Design review of the part built by this model. Coordinates are the model's own, in mm. A direction names the side the tool comes from. Give positions to 0.01 mm unless a question says otherwise; leave off trailing zeros. Order: outer loops, then holes, each group sorted by start corner. A loop starts at its lowest first (then second) coordinate and runs counter-clockwise, first axis right, second up.
```python
from build123d import *

# Parameters (mm, degrees)
SKETCH1_R           = 2
BOSS_EXTRUDE3_DEPTH = 12
CHAMFER2_SIZE       = 0.5
CUT_EXTRUDE1_DEPTH  = 2


with BuildPart() as part:
    # Sketch1 → Boss-Extrude3 (new body)
    with BuildSketch(Plane(origin=(0, 0, 0), x_dir=(1, 0, 0), z_dir=(0, 1, 0))):
        Circle(SKETCH1_R)
    extrude(amount=-BOSS_EXTRUDE3_DEPTH)

    # Sketch3 → Revolve2 (revolve)
    with BuildSketch(Plane.XY):
        with BuildLine():
            Line((-2, 0), (0, 0))
            Line((0, 0), (0, 2))
            Line((0, 2), (-3.517157288, 2))
            ThreePointArc((-3.517157288, 2), (-3.701933194, 1.876536686), (-3.658578644, 1.658578644))
            Line((-3.658578644, 1.658578644), (-2, 0))
        make_face()
    revolve(axis=Axis((0, -2, 0), (0, 1, 0)))

    # Chamfer2
    chamfer2_edges = [part.edges().sort_by_distance(p)[0] for p in [
        (-2, -12, 0),
    ]]
    chamfer(chamfer2_edges, length=CHAMFER2_SIZE)

    # Sketch4 → Cut-Extrude1 (cut)
    with BuildSketch(Plane(origin=(0, 2, 0), x_dir=(1, 0, 0), z_dir=(0, 1, 0))):
        Polygon((1.303085549, -1.141038146), (1.639710796, 0.557986116), (0.336625247, 1.699024262), (-1.303085549, 1.141038146), (-1.639710796, -0.557986116), (-0.336625247, -1.699024262), align=None)
    extrude(amount=-CUT_EXTRUDE1_DEPTH, mode=Mode.SUBTRACT)


solid = part.part
```
1. Take a section at B-B (z = 0). State the section outline as (x, y) points, then the cut area to 3 significant figures.
Recorded:
outline: (-3.66, 1.66) - (-2, 0) - (-2, -11.5) - (-1.5, -12) - (1.5, -12) - (2, -11.5) - (2, 0) - (3.66, 1.66) arc R0.2 ccw to (3.52, 2) - (1.53, 2) - (1.53, 0) - (-1.53, 0) - (-1.53, 2) - (-3.52, 2) arc R0.2 ccw to start
area: 53.5 mm2
2. For pin 1 (2 mm diameter, centred on y = -4, z = 2.5, fed in from +X); pin 2 (4 mm diameter, centred on x = 3, y = -2.5, fed in from -Z); pin 3 (4 mm diameter, centred on y = -4.5, z = 2, fed in from +X), all flat-tipped, find the tip position at first contact; note any pin that passes through.
Recorded:
pin 1: stops at x = 1.32
pin 2: stops at z = -1.73
pin 3: stops at x = 2
3. For line 1 along X through (y, z) = (-10, 0); line 2 along Y through (x, z) = (0, 0.25); line 3 along X through (y, z) = (-5.25, 0.75), list the stretches that pass through material, from the lowest coordinate up.
Recorded:
line 1: x = -2 to 2
line 2: y = -12 to 0
line 3: x = -1.85 to 1.85
4. Draft analysis for pull direction X (two halves, no side actions). For faces 3 (the face through (0, 0, 0)), 4 (the face through (0, -6, 2)), 5 (the face through (0, -12, 0)), state which applies: pulls with the +X half, pulls with the -X half, needs draft (parallel to the pull), parting line crosses it, or undercut.
Recorded:
face 3: undercut
face 4: parting line crosses it
face 5: needs draft
5. Take a section at A-A (x = 0). State the section outline as (y, z) points.
Recorded:
outline: (-12, -1.5) - (-11.5, -2) - (0, -2) - (1.66, -3.66) arc R0.2 ccw to (2, -3.52) - (2, -1.58) - (0, -1.58) - (0, 1.58) - (2, 1.58) - (2, 3.52) arc R0.2 ccw to (1.66, 3.66) - (0, 2) - (-11.5, 2) - (-12, 1.5) - close
6. Take a section at C-C (y = -2). State the section outline as (x, z) points, then the cut area to 3 significant figures.
Recorded:
outline: circle Ø4 at (0, 0)
area: 12.6 mm2
7. Machinability: for faces 1 (the face through (1.47, 1.01, 0.3)), 2 (the face through (2, 2, -1)), which of the approach directions +Z, -Z, +X, -X, +Y, -Y give a long, thin tool a straight path to every point of the face, cutting with its end or side? Answer none if there is none.
Recorded:
face 1: +Y
face 2: +Z, -Z, +X, -X, +Y
